The model under review builds one solid part; all positions refer to its coordinate system, in mm. Face numbers are marked on the shaded views. A direction names the side the tool comes from. Round coordinates to 2 decimals unless told otherwise and drop trailing zeros. Order: outer loops, then holes, each group sorted by start corner. A loop starts at its lowest first (then second) coordinate and runs counter-clockwise, first axis right, second up.
1) Consider section D-D (z = -2). Give the boundary of the cut face in (x, y), then the cut area to 3 significant figures.
2) Clearance check with flat-ended pins moving along their axes: P1, Ø1.2, axis at y = 3, z = 1.5, coming from the -X side; P2, Ø1.5, axis at x = 7.5, y = 2.5, coming from the -Z side; P3, Ø1.2, axis at x = -7.5, y = 1, coming from the -Z side. State where each tip first meets the part, or that it passes through.
3) Consider section B-B (x = 8.75). Give the boundary of the cut face in (y, z), then the cut area to 3 significant figures.
4) To check wall thickness, follow L1, parallel to Z at x = 6, y = 1.25; L2, parallel to Z at x = 5, y = 1.7; L3, parallel to Z at x = -6.5, y = 1.15. State the ranges of each line that lie inside material, in increasing order.
5) Machinability: for the marked faces 1, 2 and 3, which of the approach directions +Z, -Z, +X, -X, +Y, -Y give a long, thin tool a straight path to every point of the face, cutting with its end or side? Answer none if there is none.
6) Mouldability with a two-part tool opening along Y and no side actions: class the marked faces 4, 5, 6 and 7 as pulls with the +Y half, pulls with the -Y half, needs draft (parallel to the pull), parting line crosses it, or undercut.
7) Consider section C-C (y = 2). Give the number of separate pieces and of enclosed holes in the cut face, then the cut area to 3 significant figures.
8) Consider section A-A (z = -10.25). Give the boundary of the cut face in (x, y), then the cut area to 3 significant figures.
from build123d import *

# Parameters (mm, degrees)
SKETCH1_R               = 2.5
BOSS_EXTRUDE1_DEPTH     = 4
CUT_EXTRUDE1_DEPTH      = 23.69985803
CUT_EXTRUDE1_DEPTH_BACK = 23.69985803
SKETCH2_R               = 1.5
CUT_EXTRUDE2_START      = -6
SKETCH2_3_R             = 1.5
CUT_EXTRUDE2_DEPTH      = 17.69985803


with BuildPart() as part:
    # Sketch1 → Boss-Extrude1 (new body)
    with BuildSketch(Plane(origin=(0, 0, 0), x_dir=(1, 0, 0), z_dir=(0, 1, 0))):
        with BuildLine():
            Line((-3.917235504, 5.608829899), (-11.340461202, 5.608829899))
            Line((-11.340461202, 5.608829899), (-11.340461202, 1.608829899))
            Line((-11.340461202, 1.608829899), (-0.381690636, 1.608829899))
            Line((-0.381690636, 1.608829899), (-0.381690636, -4.391170101))
            Line((-0.381690636, -4.391170101), (-11.340461202, -4.391170101))
            Line((-11.340461202, -4.391170101), (-11.340461202, -8.391170101))
            Line((-11.340461202, -8.391170101), (4.664608782, -8.391170101))
            Line((4.664608782, -8.391170101), (13.638576545, 4.87022374))
            ThreePointArc((13.638576545, 4.87022374), (8.491842548, 16.373540203), (-1.434104983, 8.608829899))
            add(Edge.make_bspline(
                [(-1.434104983, 8.608829899), (-1.198427894, 7.122985203), (-2.407634222, 5.627246583), (-3.917235504, 5.608829899)],
                knots=[0.869474373, 0.869474373, 0.869474373, 0.869474373, 1.869474373, 1.869474373, 1.869474373, 1.869474373], degree=3))
        make_face()
        with Locations(Location((6.565895017, 8.608829899, 0), (0, 0, 270))):
            Circle(SKETCH1_R, mode=Mode.SUBTRACT)
    extrude(amount=BOSS_EXTRUDE1_DEPTH)

    # Sketch2 → Cut-Extrude1 (cut, two sides: drawn at the far end of the back side and taken through both)
    with BuildSketch(Plane.ZY.offset(0.381690636).offset(-CUT_EXTRUDE1_DEPTH_BACK)):
        with Locations((1.391170101, 2)):
            Circle(SKETCH2_R)
    extrude(amount=CUT_EXTRUDE1_DEPTH + CUT_EXTRUDE1_DEPTH_BACK, mode=Mode.SUBTRACT)

    # Sketch2<3> → Cut-Extrude2 (cut, through all)
    with BuildSketch(Plane.ZY.offset(0.381690636).offset(CUT_EXTRUDE2_START)):
        Polygon((-1.608829899, 3.732050808), (-1.608829899, 0.267949192), (1.391170101, -1.464101615), (4.391170101, 0.267949192), (4.391170101, 3.732050808), (1.391170101, 5.464101615), align=None)
        with Locations((1.391170101, 2)):
            Circle(SKETCH2_3_R, mode=Mode.SUBTRACT)
    extrude(amount=-CUT_EXTRUDE2_DEPTH, mode=Mode.SUBTRACT)


solid = part.part
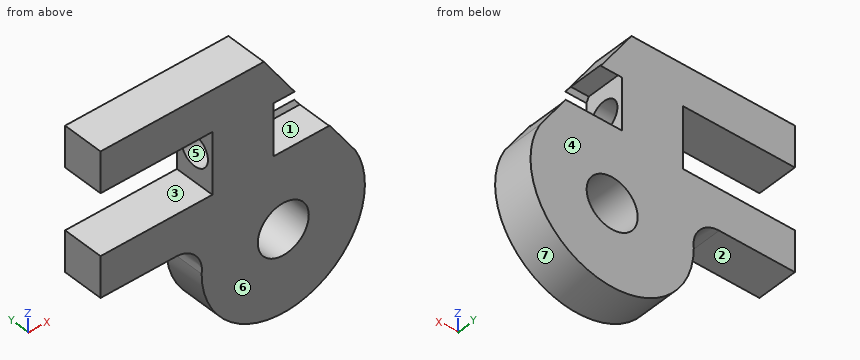
Answer below:
1. outline: (-11.34, 0) - (11.7, 0) - (11.7, 4) - (-11.34, 4) - close
1. area: 92.1 mm2
2. P1: stops at x = -0.38
2. P2: stops at z = -16.61
2. P3: stops at z = -5.61
3. outline: (0, -16.3) - (4, -16.3) - (4, -9.83) - (0, -9.83) - close; (0, -7.39) - (4, -7.39) - (4, -1.14) - (3.73, -1.61) - (0.27, -1.61) - (0, -1.14) - close
3. area: 49.2 mm2
4. L1: z = -16.59 to -11.04, -6.17 to -1.61, 4.39 to 6.42
4. L2: z = -16.45 to -10.56, -6.66 to -0.08, 2.86 to 7.9
4. L3: z = -5.61 to -1.61, 4.39 to 8.39
5. face 1: +X
5. face 2: -Z, -X, +Y, -Y
5. face 3: -X, +Y, -Y
6. face 4: pulls with the +Y half
6. face 5: undercut
6. face 6: pulls with the -Y half
6. face 7: needs draft
7. separate pieces: 2
7. enclosed holes: 1
7. area: 314 mm2
8. outline: (-1.26, 0) - (4.68, 0) - (4.68, 4) - (-1.26, 4) - close; (8.45, 0) - (14.4, 0) - (14.4, 4) - (8.45, 4) - close
8. area: 47.6 mm2
